from build123d import *

# Parameters (mm, degrees)
ESQUISSE2_W             = 650
ESQUISSE2_H             = 400
BOSS_EXTRU_1_DEPTH      = 5
ESQUISSE3_W             = 80
ESQUISSE3_H             = 40
BOSS_EXTRU_3_DEPTH      = 100
CONG_2_RADIUS           = 40
CONG_2_LENGTH           = 40
CONG_3_RADIUS           = 40
CONG_3_LENGTH           = 40
CONG_4_RADIUS           = 40
CONG_4_LENGTH           = 40
ESQUISSE6_R             = 10
ENL_V_MAT_EXTRU_2_DEPTH = 463.932230461
ESQUISSE7_R             = 10
ENL_V_MAT_EXTRU_3_DEPTH = 463.932230461
ESQUISSE9_W             = 80
ESQUISSE9_H             = 25
BOSS_EXTRU_4_DEPTH      = 49
ESQUISSE10_W            = 10.1
ESQUISSE10_H            = 3.4
BOSS_EXTRU_5_DEPTH      = 26
ENL_V_MAT_EXTRU_4_REACH = 518.908
ESQUISSE11_R            = 1.5
ESQUISSE12_W            = 10.1
ESQUISSE12_H            = 3.5
BOSS_EXTRU_6_DEPTH      = 21.6
ESQUISSE13_W            = 10.1
ESQUISSE13_H            = 2.8
BOSS_EXTRU_7_DEPTH      = 26
ENL_V_MAT_EXTRU_5_REACH = 500.416
ESQUISSE14_R            = 1.5
ESQUISSE15_W            = 5
ESQUISSE15_H            = 5
BOSS_EXTRU_8_DEPTH      = 13.75
ESQUISSE16_R            = 1.4
ENL_V_MAT_EXTRU_6_DEPTH = 513.19614407
ESQUISSE17_W            = 40
ESQUISSE17_H            = 20
BOSS_EXTRU_9_DEPTH      = 110
ESQUISSE18_W            = 40
ESQUISSE18_H            = 6
BOSS_EXTRU_10_DEPTH     = 25
ESQUISSE20_W            = 60
ESQUISSE20_H            = 40
BOSS_EXTRU_11_DEPTH     = 175.7
BOSS_EXTRU_12_REACH     = 463.014
ESQUISSE21_W            = 60
ESQUISSE21_H            = 14.1
ENL_V_MAT_EXTRU_7_REACH = 426.393
ESQUISSE22_W            = 60
ESQUISSE22_H            = 50


with BuildPart() as part:
    # Esquisse2 → Boss.-Extru.1 (new, symmetric)
    with BuildSketch(Plane(origin=(0, 0, 0), x_dir=(1, 0, 0), z_dir=(0, 1, 0))):
        Rectangle(ESQUISSE2_W, ESQUISSE2_H)
    extrude(amount=BOSS_EXTRU_1_DEPTH, both=True)

    # Esquisse3 → Boss.-Extru.3 (add)
    with BuildSketch(Plane(origin=(0, 5, 0), x_dir=(1, 0, 0), z_dir=(0, 1, 0))):
        with Locations((-235, -92.5)):
            Rectangle(ESQUISSE3_W, ESQUISSE3_H)
        with Locations((235, 92.5)):
            Rectangle(ESQUISSE3_W, ESQUISSE3_H)
        with Locations((-235, 92.5)):
            Rectangle(ESQUISSE3_W, ESQUISSE3_H)
    extrude(amount=BOSS_EXTRU_3_DEPTH)

    # Congé2: full round fillet: the end face becomes a half cylinder, R = half its width
    cong_2_face = Plane((-235, 105, 92.5), x_dir=(0, 0, -1), z_dir=(0, 1, 0))  # on the end face: x along it, z out of the body
    cong_2_slab = cong_2_face.offset(-CONG_2_RADIUS / 2) * Box(CONG_2_LENGTH, 2 * CONG_2_RADIUS, CONG_2_RADIUS, mode=Mode.PRIVATE)  # the body's end, R deep
    cong_2_round = Plane((-235, 65, 92.5), x_dir=(0, 1, 0), z_dir=(0, 0, -1)) * Cylinder(CONG_2_RADIUS, CONG_2_LENGTH, mode=Mode.PRIVATE)  # its axis R under the face
    add(cong_2_slab - cong_2_round, mode=Mode.SUBTRACT)

    # Congé3: full round fillet: the end face becomes a half cylinder, R = half its width
    cong_3_face = Plane((-235, 105, -92.5), x_dir=(0, 0, -1), z_dir=(0, 1, 0))  # on the end face: x along it, z out of the body
    cong_3_slab = cong_3_face.offset(-CONG_3_RADIUS / 2) * Box(CONG_3_LENGTH, 2 * CONG_3_RADIUS, CONG_3_RADIUS, mode=Mode.PRIVATE)  # the body's end, R deep
    cong_3_round = Plane((-235, 65, -92.5), x_dir=(0, 1, 0), z_dir=(0, 0, -1)) * Cylinder(CONG_3_RADIUS, CONG_3_LENGTH, mode=Mode.PRIVATE)  # its axis R under the face
    add(cong_3_slab - cong_3_round, mode=Mode.SUBTRACT)

    # Congé4: full round fillet: the end face becomes a half cylinder, R = half its width
    cong_4_face = Plane((235, 105, -92.5), x_dir=(0, 0, -1), z_dir=(0, 1, 0))  # on the end face: x along it, z out of the body
    cong_4_slab = cong_4_face.offset(-CONG_4_RADIUS / 2) * Box(CONG_4_LENGTH, 2 * CONG_4_RADIUS, CONG_4_RADIUS, mode=Mode.PRIVATE)  # the body's end, R deep
    cong_4_round = Plane((235, 65, -92.5), x_dir=(0, 1, 0), z_dir=(0, 0, -1)) * Cylinder(CONG_4_RADIUS, CONG_4_LENGTH, mode=Mode.PRIVATE)  # its axis R under the face
    add(cong_4_slab - cong_4_round, mode=Mode.SUBTRACT)

    # Esquisse6 → Enlèv. mat.-Extru.2 (cut, through all)
    with BuildSketch(Plane.XY.offset(112.5)):
        with Locations((-235, 63)):
            Circle(ESQUISSE6_R)
    extrude(amount=-ENL_V_MAT_EXTRU_2_DEPTH, mode=Mode.SUBTRACT)

    # Esquisse7 → Enlèv. mat.-Extru.3 (cut, through all)
    with BuildSketch(Plane(origin=(0, 0, -112.5), x_dir=(-1, 0, 0), z_dir=(0, 0, -1))):
        with Locations((-235, 63)):
            Circle(ESQUISSE7_R)
    extrude(amount=-ENL_V_MAT_EXTRU_3_DEPTH, mode=Mode.SUBTRACT)

    # Esquisse9 → Boss.-Extru.4 (add)
    with BuildSketch(Plane(origin=(0, 5, 0), x_dir=(1, 0, 0), z_dir=(0, 1, 0))):
        with Locations((100, -175.5)):
            Rectangle(ESQUISSE9_W, ESQUISSE9_H)
    extrude(amount=BOSS_EXTRU_4_DEPTH)

    # Esquisse10 → Boss.-Extru.5 (add)
    with BuildSketch(Plane(origin=(0, 54, 0), x_dir=(1, 0, 0), z_dir=(0, 1, 0))):
        with Locations((105.62, -186.3)):
            Rectangle(ESQUISSE10_W, ESQUISSE10_H)
    extrude(amount=BOSS_EXTRU_5_DEPTH)

    # Esquisse11 → Enlèv. mat.-Extru.4 (cut, up to next)
    with BuildSketch(Plane.XY.offset(188), mode=Mode.PRIVATE) as enl_v_mat_extru_4_sk1:
        with Locations((105.62, 56.5)):
            Circle(ESQUISSE11_R)
    enl_v_mat_extru_4_tool1 = extrude(enl_v_mat_extru_4_sk1.sketch, amount=-ENL_V_MAT_EXTRU_4_REACH, mode=Mode.PRIVATE) & part.part
    # Esquisse11 → Enlèv. mat.-Extru.4 (cut, up to next)
    with BuildSketch(Plane.XY.offset(188), mode=Mode.PRIVATE) as enl_v_mat_extru_4_sk2:
        with Locations((105.62, 74)):
            Circle(ESQUISSE11_R)
    enl_v_mat_extru_4_tool2 = extrude(enl_v_mat_extru_4_sk2.sketch, amount=-ENL_V_MAT_EXTRU_4_REACH, mode=Mode.PRIVATE) & part.part
    add(enl_v_mat_extru_4_tool1.solids().sort_by_distance((105.62, 56.5, 188))[0], mode=Mode.SUBTRACT)
    add(enl_v_mat_extru_4_tool2.solids().sort_by_distance((105.62, 74, 188))[0], mode=Mode.SUBTRACT)

    # Esquisse12 → Boss.-Extru.6 (add)
    with BuildSketch(Plane(origin=(0, 0, 184.6), x_dir=(-1, 0, 0), z_dir=(0, 0, -1))):
        with Locations((-105.62, 78.25)):
            Rectangle(ESQUISSE12_W, ESQUISSE12_H)
    extrude(amount=BOSS_EXTRU_6_DEPTH)

    # Esquisse13 → Boss.-Extru.7 (add)
    with BuildSketch(Plane(origin=(0, 80, 0), x_dir=(1, 0, 0), z_dir=(0, 1, 0))):
        with Locations((105.62, -164.4)):
            Rectangle(ESQUISSE13_W, ESQUISSE13_H)
    extrude(amount=-BOSS_EXTRU_7_DEPTH)

    # Esquisse14 → Enlèv. mat.-Extru.5 (cut, up to next)
    with BuildSketch(Plane(origin=(0, 0, 163), x_dir=(-1, 0, 0), z_dir=(0, 0, -1)), mode=Mode.PRIVATE) as enl_v_mat_extru_5_sk1:
        with Locations(Location((-105.62, 74, 0), (0, 0, 180))):
            Circle(ESQUISSE14_R)
    enl_v_mat_extru_5_tool1 = extrude(enl_v_mat_extru_5_sk1.sketch, amount=-ENL_V_MAT_EXTRU_5_REACH, mode=Mode.PRIVATE) & part.part
    # Esquisse14 → Enlèv. mat.-Extru.5 (cut, up to next)
    with BuildSketch(Plane(origin=(0, 0, 163), x_dir=(-1, 0, 0), z_dir=(0, 0, -1)), mode=Mode.PRIVATE) as enl_v_mat_extru_5_sk2:
        with Locations(Location((-105.62, 56.5, 0), (0, 0, 180))):
            Circle(ESQUISSE14_R)
    enl_v_mat_extru_5_tool2 = extrude(enl_v_mat_extru_5_sk2.sketch, amount=-ENL_V_MAT_EXTRU_5_REACH, mode=Mode.PRIVATE) & part.part
    add(enl_v_mat_extru_5_tool1.solids().sort_by_distance((105.62, 74, 163))[0], mode=Mode.SUBTRACT)
    add(enl_v_mat_extru_5_tool2.solids().sort_by_distance((105.62, 56.5, 163))[0], mode=Mode.SUBTRACT)

    # Esquisse15 → Boss.-Extru.8 (add)
    with BuildSketch(Plane(origin=(0, 54, 0), x_dir=(1, 0, 0), z_dir=(0, 1, 0))):
        with Locations((71.32, -179.2)):
            Rectangle(ESQUISSE15_W, ESQUISSE15_H)
        with Locations((71.32, -171.2)):
            Rectangle(ESQUISSE15_W, ESQUISSE15_H)
    extrude(amount=BOSS_EXTRU_8_DEPTH)

    # Esquisse16 → Enlèv. mat.-Extru.6 (cut, through all)
    with BuildSketch(Plane.XY.offset(181.7)):
        with Locations((71.22, 65.25)):
            Circle(ESQUISSE16_R)
    enl_v_mat_extru_6 = extrude(amount=-ENL_V_MAT_EXTRU_6_DEPTH, mode=Mode.SUBTRACT)

    # Esquisse17 → Boss.-Extru.9 (add)
    with BuildSketch(Plane(origin=(0, 5, 0), x_dir=(1, 0, 0), z_dir=(0, 1, 0))):
        with Locations((-155, -82.5)):
            Rectangle(ESQUISSE17_W, ESQUISSE17_H)
        with Locations((-155, 82.5)):
            Rectangle(ESQUISSE17_W, ESQUISSE17_H)
    boss_extru_9 = extrude(amount=BOSS_EXTRU_9_DEPTH)

    # Esquisse18 → Boss.-Extru.10 (add)
    with BuildSketch(Plane(origin=(0, 115, 0), x_dir=(1, 0, 0), z_dir=(0, 1, 0))):
        with Locations((-155, 82.5)):
            Rectangle(ESQUISSE18_W, ESQUISSE18_H)
    boss_extru_10 = extrude(amount=BOSS_EXTRU_10_DEPTH)

    # Esquisse20 → Boss.-Extru.11 (add)
    with BuildSketch(Plane(origin=(0, 5, 0), x_dir=(1, 0, 0), z_dir=(0, 1, 0))):
        with Locations((-80.1874064, -92.5)):
            Rectangle(ESQUISSE20_W, ESQUISSE20_H)
        with Locations((-80.1874064, 92.5)):
            Rectangle(ESQUISSE20_W, ESQUISSE20_H)
    extrude(amount=BOSS_EXTRU_11_DEPTH)

    # Esquisse21 → Boss.-Extru.12 (add, up to next)
    with BuildSketch(Plane.XY.offset(-72.5), mode=Mode.PRIVATE) as boss_extru_12_sk1:
        with Locations((-80.1874064, 173.65)):
            Rectangle(ESQUISSE21_W, ESQUISSE21_H)
    boss_extru_12_tool1 = extrude(boss_extru_12_sk1.sketch, amount=BOSS_EXTRU_12_REACH, mode=Mode.PRIVATE) - part.part
    add(boss_extru_12_tool1.solids().sort_by_distance((-80.187406, 173.65, -72.5))[0])

    # Esquisse22 → Enlèv. mat.-Extru.7 (cut, up to next)
    with BuildSketch(Plane(origin=(0, 180.7, 0), x_dir=(1, 0, 0), z_dir=(0, 1, 0)), mode=Mode.PRIVATE) as enl_v_mat_extru_7_sk1:
        with Locations((-80.1874064, 0)):
            Rectangle(ESQUISSE22_W, ESQUISSE22_H)
    enl_v_mat_extru_7_tool1 = extrude(enl_v_mat_extru_7_sk1.sketch, amount=-ENL_V_MAT_EXTRU_7_REACH, mode=Mode.PRIVATE) & part.part
    add(enl_v_mat_extru_7_tool1.solids().sort_by_distance((-80.187406, 180.7, 0))[0], mode=Mode.SUBTRACT)

    # Symétrie1: Enlèv. mat.-Extru.6, Boss.-Extru.9, Boss.-Extru.10 across plane
    add(enl_v_mat_extru_6.mirror(Plane(origin=(0, 0, 0), x_dir=(0, 0, 1), z_dir=(1, 0, 0))), mode=Mode.SUBTRACT)
    add(boss_extru_9.mirror(Plane(origin=(0, 0, 0), x_dir=(0, 0, 1), z_dir=(1, 0, 0))))
    add(boss_extru_10.mirror(Plane(origin=(0, 0, 0), x_dir=(0, 0, 1), z_dir=(1, 0, 0))))


solid = part.part
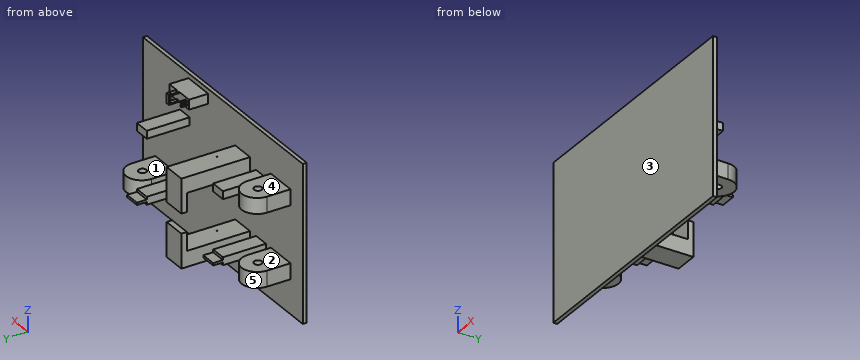
Geometry: final body of the model. Coordinates: model frame, mm. Face numbers are marked on the shaded views. A direction names the side the tool comes from. Give positions to 0.01 mm unless a question says otherwise; leave off trailing zeros. Write each loop counter-clockwise with the first axis right and the second up, starting at its lowest first coordinate (ties: lowest second). Pieces come first, ordered by that corner, then holes. Notation, with made-up numbers: (-21, -1.75) -> (23, -1.75) arc R26 cw to (23, 25.25) -> close; hole circle Ø10 at (-19, -33). An arc over 180 degrees is marked (long way). Answer as a JSON object with one key per item and string values.
1. Cut plane D-D on x = -80.5. Output: boundary loops of the cut face in (y, z), and give its area (3 significant figures).
Ans:
{"outline": "(-5, -200) -> (5, -200) -> (5, -112.5) -> (180.7, -112.5) -> (180.7, -25) -> (166.6, -25) -> (166.6, -72.5) -> (5, -72.5) -> (5, 72.5) -> (166.6, 72.5) -> (166.6, 25) -> (180.7, 25) -> (180.7, 112.5) -> (5, 112.5) -> (5, 200) -> (-5, 200) -> close", "area": "19,400 mm^2"}
2. Cut plane A-A on x = 235. Output: boundary loops of the cut face in (y, z).
Ans:
{"outline": "(-5, -200) -> (5, -200) -> (5, -112.5) -> (53, -112.5) -> (53, -72.5) -> (5, -72.5) -> (5, 200) -> (-5, 200) -> close; (73, -112.5) -> (105, -112.5) -> (105, -72.5) -> (73, -72.5) -> close"}
3. Cut plane B-B on x = -235. Output: boundary loops of the cut face in (y, z), and give its area (3 significant figures).
Ans:
{"outline": "(-5, -200) -> (5, -200) -> (5, -112.5) -> (53, -112.5) -> (53, -72.5) -> (5, -72.5) -> (5, 72.5) -> (53, 72.5) -> (53, 112.5) -> (5, 112.5) -> (5, 200) -> (-5, 200) -> close; (73, -112.5) -> (105, -112.5) -> (105, -72.5) -> (73, -72.5) -> close; (73, 72.5) -> (105, 72.5) -> (105, 112.5) -> (73, 112.5) -> close", "area": "10,400 mm^2"}
4. Contact query for flat-ended pins moving along their axis: pin 1 (6 mm diameter, centred on y = 78, z = -87, fed in from +X); pin 2 (8 mm diameter, centred on x = 106, y = 70.5, fed in from +Z); pin 3 (2 mm diameter, centred on x = -255.5, y = 58.5, fed in from -Z); pin 4 (1.8 mm diameter, centred on x = 105.62, y = 74, fed in from -Z). Output: stop coordinate, or through.
Ans:
{"pin 1": "stops at x = 273.73", "pin 2": "stops at z = 188", "pin 3": "stops at z = -112.5", "pin 4": "passes through"}
5. Ray query, probe 1 along Y at (x, z) = (105.62, 165); probe 2 along Y at (x, z) = (71.22, 179.95); probe 3 along Y at (x, z) = (-71.22, 100.5). Return the intervals inside material, ascending. Write a range as from..to.
Ans:
{"probe 1": "y = -5..55, 58..72.5, 75.5..80", "probe 2": "y = -5..63.85, 66.65..67.75", "probe 3": "y = -5..63.85, 66.65..180.7"}
6. Access query for the marked faces 4 and 5. Directions: +Z, -Z, +X, -X, +Y, -Y. A direction counts if a zero-diameter tool reaches every point of the face in a straight line with its end or side. Return the directions, or none.
Ans:
{"face 4": "+Z, +X, -X, +Y", "face 5": "+Z, -Z, +Y"}
7. Cut plane C-C on y = 160. Output: boundary loops of the cut face in (x, z), and give its area (3 significant figures).
Ans:
{"outline": "(-110.19, -112.5) -> (-50.19, -112.5) -> (-50.19, -72.5) -> (-110.19, -72.5) -> close; (-110.19, 72.5) -> (-50.19, 72.5) -> (-50.19, 112.5) -> (-110.19, 112.5) -> close", "area": "4,800 mm^2"}
8. Mould query, pull axis Z, two halves, no side actions, for the marked faces 1, 2 and 3. Classes: pulls with the +Z half, pulls with the -Z half, needs draft (parallel to the pull), parting line crosses it, or undercut.
Ans:
{"face 1": "pulls with the +Z half", "face 2": "undercut", "face 3": "needs draft"}
